Here's how the part is built. I have some questions about the finished solid (model axes, mm). Face numbers are marked on the shaded views. Round coordinates to 2 decimals unless told otherwise and drop trailing zeros. Loops run counter-clockwise (first coordinate to the right, second up) from the corner with the lowest first, then second, coordinate; pieces in that order, holes last. Notation, with made-up numbers: (23.25, 0.5) -> (48.25, 0.5) arc R26 cw to (48.25, 15.5) -> close; hole circle Ø6 at (89, 61). An arc over 180 degrees is marked (long way). Use one line per item in the form item = value. Start each with the question number.
Item 1: I'm going to push flat-ended pins straight in: pin 1 Ø3 at (y, z) = (28.5, -64) entering from +X; pin 2 Ø2 at (x, y) = (42.5, 7) entering from -Z; pin 3 Ø1.5 at (x, y) = (-17, 17.5) entering from -Z. Where does each tip first touch, or does it pass through?
Item 2: If we section it at C-C (y = 4): Write out the boundary of the cut face in (x, z).
Item 3: If we section it at A-A (z = 0): Write out the boundary of the cut face in (x, y).
Item 4: Thinking about a two-plate mould opening in X: for the marked faces 1, 2 and 3, which applies, released by +X, released by -X, zero draft, split by the parting line, or undercut?
Item 5: If we section it at B-B (x = 0): Write out the boundary of the cut face in (y, z), then the cut area to 3 significant figures.
Item 6: If I drill on L1, parallel to Z at x = 0, y = 11.5; L2, parallel to Z at x = 0, y = 6.35, over which ranges is the centre line in solid material (lowest first)? Write a range as [from, to].
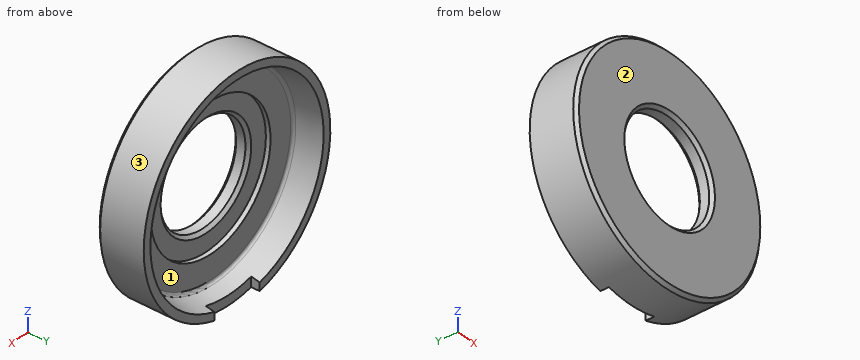
Autodesk Inventor part; units mm, degrees
ref_plane "YZ Plane" through (0, 0, 0) normal (1, 0, 0) x (0, 1, 0)
ref_plane "XZ Plane" through (0, 0, 0) normal (0, 1, 0) x (-1, 0, 0)
ref_plane "XY Plane" through (0, 0, 0) normal (0, 0, 1) x (1, 0, 0)
sketch "Эскиз1" plane through (0, 0, 0) normal (0, 0, 1) x (1, 0, 0)
  line L0 (0, 0) -> (70, 0)
  line L1 (70, 0) -> (70, 30)
  line L2 (70, 30) -> (65, 30)
  line L3 (32, 13) -> (32, 0)
  line L4 (65, 30) -> (61.7485, 13)
  line L5 (0, -6) -> (0, 36)
  line L6 (32, 13) -> (61.7485, 13)
  dimension "d0" = 70
  dimension "d1" = 30
  dimension "d2" = 5
  dimension "d16" = 32
revolve "Вращение1" add sketch "Эскиз1" angle 360 about axis through (0, -10, 0) along (0, 1, 0)
sketch "Эскиз2" plane through (0, 13, 0) normal (0, 1, 0) x (1, 0, 0)
  circle A0 centre (0, 0) radius 45
  circle A1 centre (0, 0) radius 32
  dimension "d6" = 90
extrude "Выдавливание1" cut sketch "Эскиз2" against normal blind 3
chamfer "Фаска1" distance 2 angle 45 2 edges at (-32, 10, 0) (-32, 0, 0)
chamfer "Фаска2" distance 2 angle 45 1 edges at (-70, 0, 0)
fillet "Сопряжение1" radius 2 1 edges at (-61.7485, 13, 0)
sketch "Эскиз3" plane through (0, 0, 0) normal (0, 0, 1) x (1, 0, 0)
  line L0 (0, 0) -> (0, -10)
  line L1 (-17.039, 24.5) -> (-17.039, 30)
  line L2 (17.039, 24.5) -> (-17.039, 24.5)
  line L3 (0, -18.3) -> (0, 39.8)
  line L4 (0, 30) -> (17.039, 30)
  line L5 (-70, 30) -> (70, 30)
  line L6 (17.039, 30) -> (17.039, 24.5)
  line L7 (0, 30) -> (-17.039, 30)
extrude "Выдавливание2" cut sketch "Эскиз3" against normal through all
properties part number "Корпус маслосъемника" material "Чугун, серый"
Values found:
q1.pin_1 = 31.52
q1.pin_2 = -56.37
q1.pin_3 = -68.09
q2.outline = circle Ø140 at (0, 0); hole circle Ø64 at (0, 0)
q3.outline = (-70, 2) -> (-68, 0) -> (-34, 0) -> (-32, 2) -> (-32, 8) -> (-34, 10) -> (-45, 10) -> (-45, 13) -> (-60.09, 13) arc R2 cw to (-62.06, 14.62) -> (-65, 30) -> (-70, 30) -> close; (32, 2) -> (34, 0) -> (68, 0) -> (70, 2) -> (70, 30) -> (65, 30) -> (62.06, 14.62) arc R2 cw to (60.09, 13) -> (45, 13) -> (45, 10) -> (34, 10) -> (32, 8) -> close
q4.face_1 = undercut
q4.face_2 = zero draft
q4.face_3 = split by the parting line
q5.outline = (0, -68) -> (2, -70) -> (24.5, -70) -> (24.5, -63.95) -> (14.62, -62.06) arc R2 cw to (13, -60.09) -> (13, -45) -> (10, -45) -> (10, -34) -> (8, -32) -> (2, -32) -> (0, -34) -> close; (0, 34) -> (2, 32) -> (8, 32) -> (10, 34) -> (10, 45) -> (13, 45) -> (13, 60.09) arc R2 cw to (14.62, 62.06) -> (30, 65) -> (30, 70) -> (2, 70) -> (0, 68) -> close
q5.area = 1,090 mm2
q6.L1 = [-70, -45], [45, 70]
q6.L2 = [-70, -32], [32, 70]
